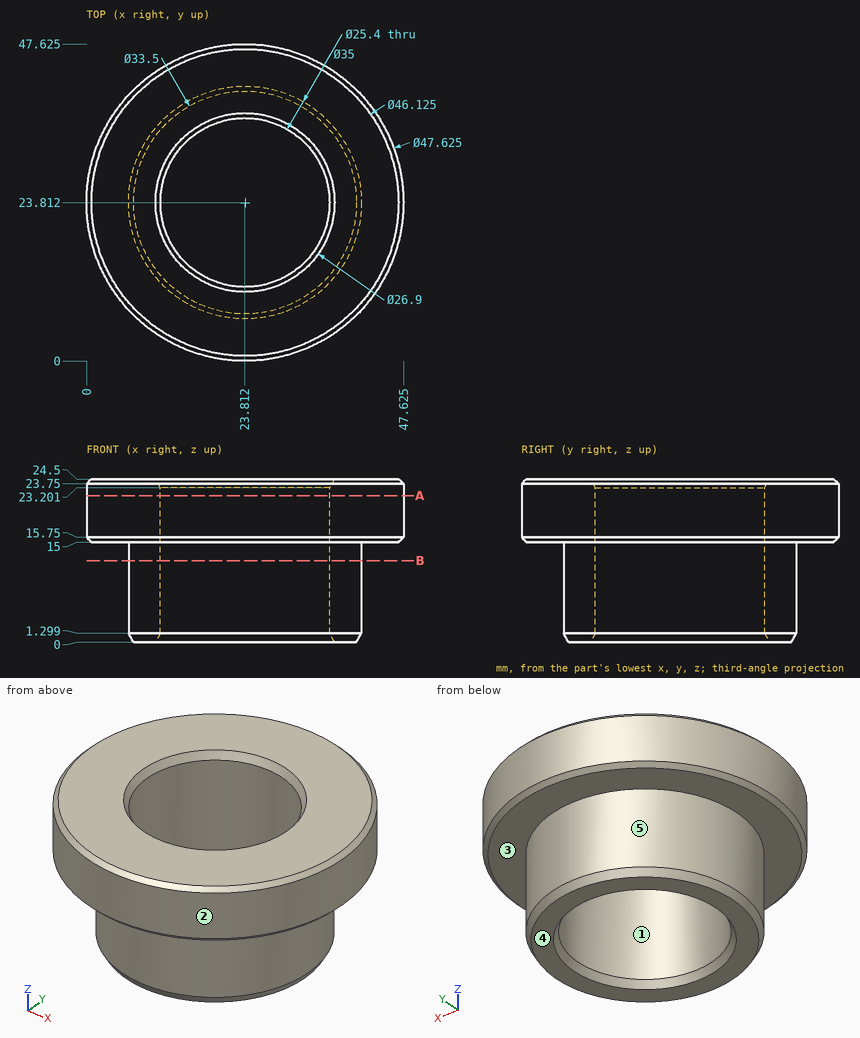
Verification items for this drawing (mm, ordinates from the low corner). A direction names the side the tool comes from. Round coordinates to 2 decimals unless told otherwise and drop trailing zeros. Loops run counter-clockwise (first coordinate to the right, second up) from the corner with the lowest first, then second, coordinate; pieces in that order, holes last. Notation, with made-up numbers: (24.25, -23) -> (66.25, -23) arc R14 ccw to (66.25, -17) -> close; hole circle Ø5 at (-4, 37). An arc over 180 degrees is marked (long way). Answer in a Markdown table with one row per item.
Q1. Thickness scan on L1, parallel to Y at x = 33.5, z = 6 (1 decimal); L2, parallel to X at y = 17, z = 7.25 (1 decimal); L3, parallel to Z at x = 20, y = 41. Record the ranges inside material, lowest first.
Data:
| item | result |
|---|---|
| L1 | y = 9.2 to 15.6, 32 to 38.4 |
| L2 | x = 7.7 to 13.1, 34.5 to 39.9 |
| L3 | z = 15 to 24.5 |
Q2. Sectioned sample at B-B on z = 12.25. Enter the section's corners in (x, y).
Data:
| item | result |
|---|---|
| outline | circle Ø35 at (23.81, 23.81); hole circle Ø25.4 at (23.81, 23.81) |
Q3. Go/stop test with flat-tipped pins: P1, Ø3, axis at x = 39.5, z = 22, coming from the +Y side; P2, Ø8, axis at y = 28, z = 8.5, coming from the -X side; P3, Ø5, axis at y = 19.5, z = 5.5, coming from the -X side. Record where each tip stops, or that it passes through.
Data:
| item | result |
|---|---|
| P1 | stops at y = 42.94 |
| P2 | stops at x = 6.31 |
| P3 | stops at x = 6.41 |
Q4. Set-up check for the marked faces 4 and 5: record each of +Z, -Z, +X, -X, +Y, -Y from which the full face is reachable in a straight line by a thin tool's end or side.
Data:
| item | result |
|---|---|
| face 4 | -Z, +X, -X, +Y, -Y |
| face 5 | -Z |
Q5. Sectioned sample at A-A on z = 22. Enter the section's corners in (x, y) (1 decimal).
Data:
| item | result |
|---|---|
| outline | circle Ø47.6 at (23.8, 23.8); hole circle Ø25.4 at (23.8, 23.8) |
Q6. Release check for a two-part mould opening along X. For the marked faces 1, 2 and 3 record: released by +X, released by -X, zero draft, split by the parting line, or undercut.
Data:
| item | result |
|---|---|
| face 1 | undercut |
| face 2 | split by the parting line |
| face 3 | zero draft |
